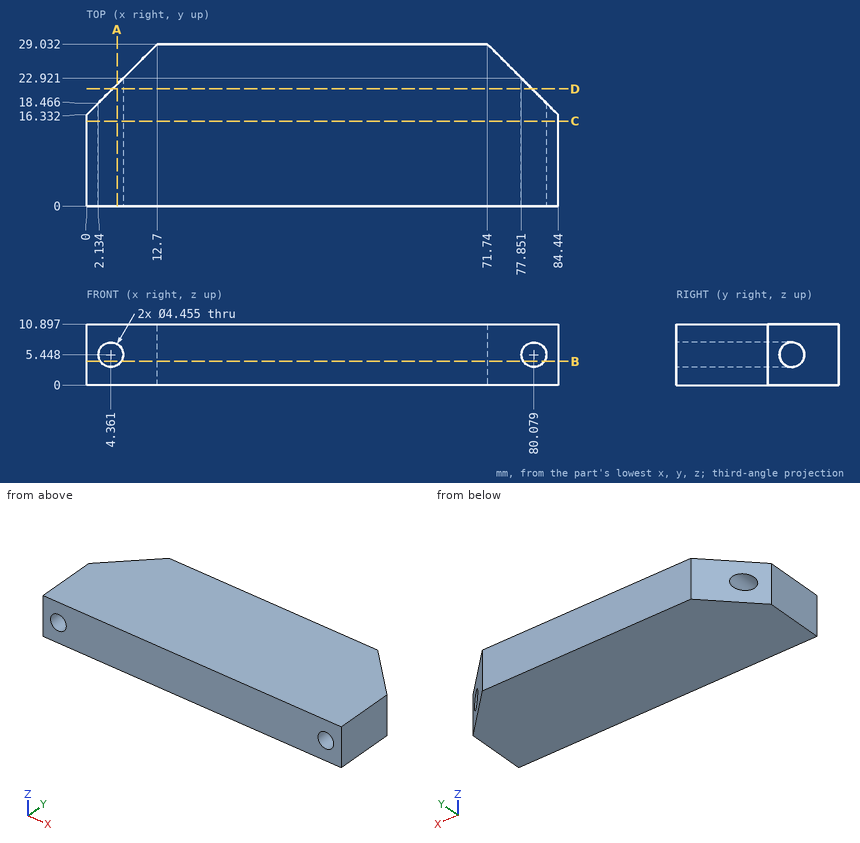
Study the drawing (mm; zero at the part's minimum x, y, z) and answer. Coordinates: 2 decimals unless noted, no trailing zeros. Loops run counter-clockwise (first coordinate to the right, second up) from the corner with the lowest first, then second, coordinate; pieces in that order, holes last. Notation, with made-up numbers: M 4,39 L 35,39 A26 ccw 35,65 Z; hole C 64,24 d11. An arc over 180 degrees is marked long. Answer in a Markdown table with one row per item. Add a question column.
1. Find section B-B, the plane z = 4.25. Write down the section's boundary in (x, y) (1 decimal), then the cut area to 3 significant figures.
2. A flat-ended cylindrical pin translates along its axis: P1, Ø6, axis at x = 4.36, z = 5.45, coming from the +Y side. Find the tip coordinate at first contact, or state that the pin passes through.
3. Find section D-D, the plane y = 21. Write down the section's boundary in (x, z) (1 decimal).
4. Find section C-C, the plane y = 15.25. Write down the section's boundary in (x, z) (1 decimal), then the cut area to 3 significant figures.
5. Consider L1, parallel to X at y = 11, z = 7 (1 decimal); L2, parallel to X at y = 12.25, z = 5.25; L3, parallel to X at y = 20, z = 1.75. Determine where each line is inside the solid, lowest interval first.
6. Find section A-A, the plane x = 5.5. Write down the section's boundary in (y, z).
Reported:
| question | item | result |
|---|---|---|
| 1 | outline | M 0,0 L 2.5,0 L 2.5,18.8 L 0,16.3 Z; M 6.2,0 L 78.2,0 L 78.2,22.6 L 71.7,29 L 12.7,29 L 6.2,22.6 Z; M 82,0 L 84.4,0 L 84.4,16.3 L 82,18.8 Z |
| 1 | area | 2,130 mm^2 |
| 2 | P1 | stops at y = 23.69 |
| 3 | outline | M 4.7,0 L 79.8,0 L 79.8,3.2 A2.2 cw 79.8,7.7 L 79.8,10.9 L 4.7,10.9 L 4.7,7.7 A2.2 cw 4.7,3.2 Z |
| 4 | outline | M 0,0 L 84.4,0 L 84.4,10.9 L 0,10.9 Z; hole C 4.4,5.4 d4.5; hole C 80.1,5.4 d4.5 |
| 4 | area | 889 mm^2 |
| 5 | L1 | x = 0 to 2.8, 6 to 78.5, 81.7 to 84.4 |
| 5 | L2 | x = 0 to 2.14, 6.58 to 77.86, 82.3 to 84.44 |
| 5 | L3 | x = 3.67 to 80.77 |
| 6 | outline | M 0,0 L 21.83,0 L 21.83,3.53 L 0,3.53 Z; M 0,7.36 L 21.83,7.36 L 21.83,10.9 L 0,10.9 Z |
